Geometry: see drawing. Coordinates: mm, zero at the bounding-box minimum. A direction names the side the tool comes from. Give positions to 0.01 mm unless a question says otherwise; leave off trailing zeros. Write each loop counter-clockwise with the first axis right and the second up, starting at its lowest first coordinate (ties: lowest second). Pieces come first, ordered by that corner, then holes. Notation, with made-up numbers: (29.25, 9) -> (47.25, 9) arc R27 ccw to (47.25, 46) -> close; hole circle Ø5 at (4.5, 44.25). An arc over 180 degrees is marked (long way). Write item = value, one per line.
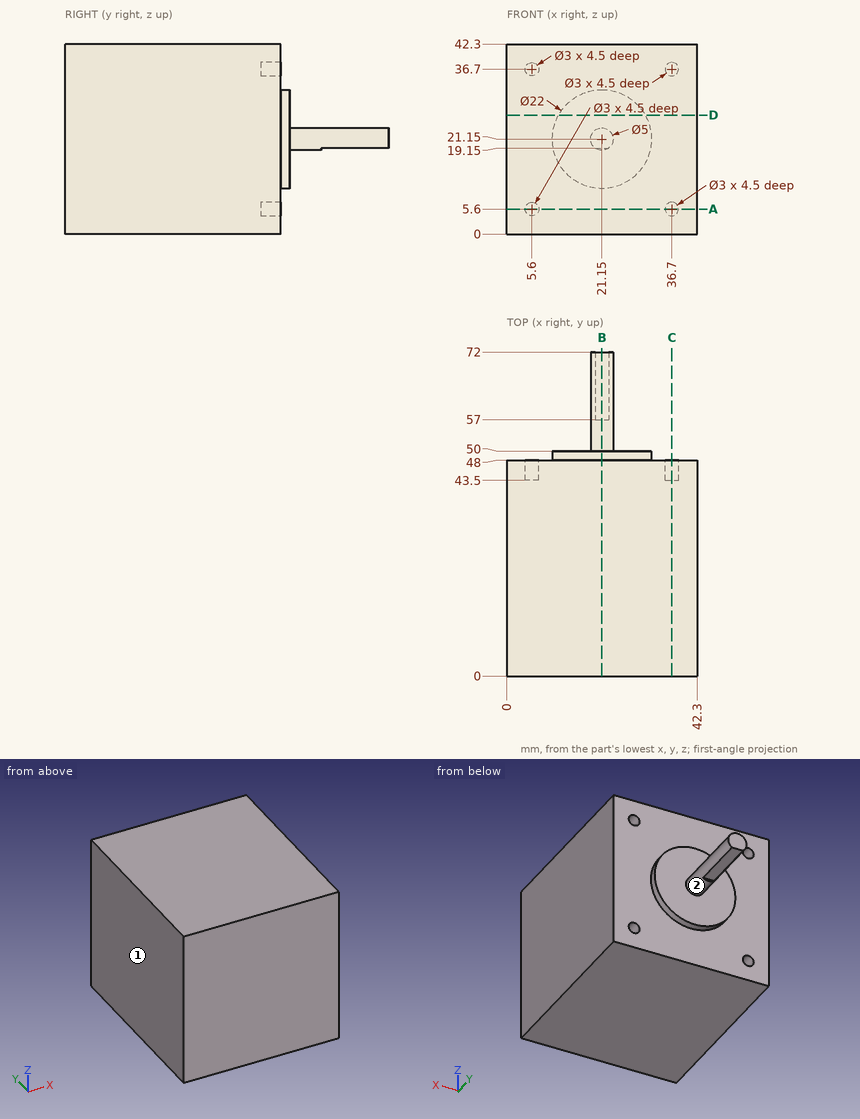
(1) Section query A-A (z = 5.6). Return loops of the section in (x, y).
Values follow:
outline = (0, 0) -> (42.3, 0) -> (42.3, 48) -> (38.2, 48) -> (38.2, 43.5) -> (35.2, 43.5) -> (35.2, 48) -> (7.1, 48) -> (7.1, 43.5) -> (4.1, 43.5) -> (4.1, 48) -> (0, 48) -> close
(2) Section query D-D (z = 26.5). Return loops of the section in (x, y), plus the area to 3 significant figures.
Values follow:
outline = (0, 0) -> (42.3, 0) -> (42.3, 48) -> (30.76, 48) -> (30.76, 50) -> (11.54, 50) -> (11.54, 48) -> (0, 48) -> close
area = 2,070 mm2
(3) Section query C-C (x = 36.7). Return loops of the section in (y, z), plus the area to 3 significant figures.
Values follow:
outline = (0, 0) -> (48, 0) -> (48, 4.1) -> (43.5, 4.1) -> (43.5, 7.1) -> (48, 7.1) -> (48, 35.2) -> (43.5, 35.2) -> (43.5, 38.2) -> (48, 38.2) -> (48, 42.3) -> (0, 42.3) -> close
area = 2,000 mm2
(4) First-contact query: pin 1 (2.5 mm diameter, centred on x = 20.5, y = 61, fed in from -Z); pin 2 (6 mm diameter, centred on x = 25.5, z = 25, fed in from +Y); pin 3 (1.5 mm diameter, centred on x = 37, z = 5, fed in from +Y). Flat tips, straight axial feed; report the tip coordinate or a pass-through.
Values follow:
pin_1 = 19.15
pin_2 = 50
pin_3 = 43.5
(5) Access query for the marked faces 1 and 2. Directions: +Z, -Z, +X, -X, +Y, -Y. A direction counts if a zero-diameter tool reaches every point of the face in a straight line with its end or side. Return the directions, or none.
Values follow:
face_1 = +Z, -Z, -X, +Y, -Y
face_2 = +Y
(6) Material intervals for line 1 (X direction, y = 45.9, z = 5.6); line 2 (X direction, y = 44, z = 36), sorted ascending.
Values follow:
line_1 = 0 to 4.1, 7.1 to 35.2, 38.2 to 42.3
line_2 = 0 to 4.27, 6.93 to 35.37, 38.03 to 42.3
(7) Section query B-B (x = 21.15). Return loops of the section in (y, z).
Values follow:
outline = (0, 0) -> (48, 0) -> (48, 10.15) -> (50, 10.15) -> (50, 18.65) -> (57, 18.65) -> (57, 19.15) -> (72, 19.15) -> (72, 23.65) -> (50, 23.65) -> (50, 32.15) -> (48, 32.15) -> (48, 42.3) -> (0, 42.3) -> close
